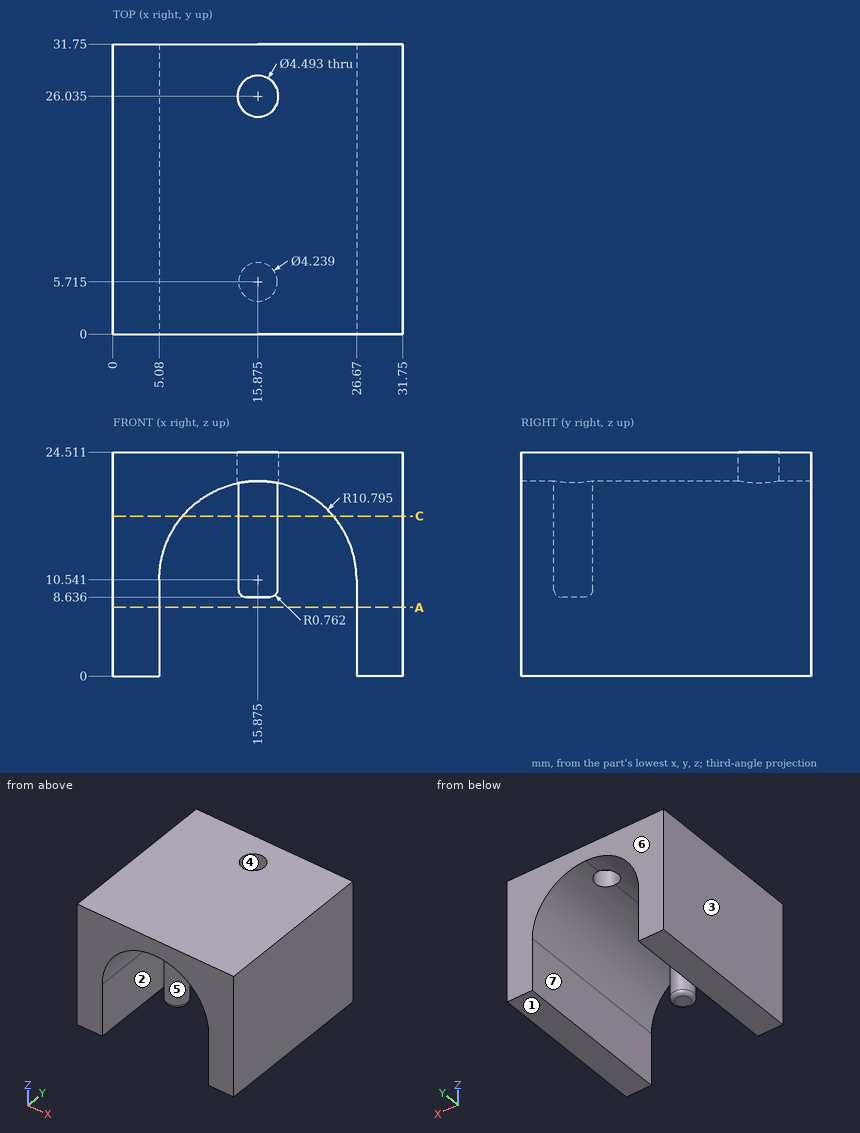
For this review, use the dimensioned drawing (mm, ordinates from the lowest corner) and the shaded views. A direction names the side the tool comes from. Give positions to 0.01 mm unless a question says otherwise; leave off trailing zeros. Write each loop counter-clockwise with the first axis right and the second up, starting at its lowest first coordinate (ties: lowest second). Pieces come first, ordered by that corner, then holes.
(1) Tool access review of the marked faces 5, 6 and 7: name each direction out of +Z, -Z, +X, -X, +Y, -Y from which nothing blocks a thin tool from reaching the whole face with its end or side.
(2) The part is to be moulded in two halves that separate along X. For the marked faces 1, 2, 3 and 4, say which applies: released by +X, released by -X, zero draft, split by the parting line, or undercut.
(3) Consider section A-A, the plane z = 7.5. Give the boundary of the cut face in (x, y).
(4) Consider section C-C, the plane z = 17.5. Give the number of separate pieces and of enclosed holes in the cut face, and give its area (3 significant figures).
(5) For P1, Ø1.5, axis at y = 18, z = 21.5, coming from the -X side; P2, Ø0.8, axis at x = 16, y = 6, coming from the -Z side; P3, Ø10, axis at x = 12.5, z = 14, coming from the -Y side, all flat-tipped, find the tip position at first contact; note any pin that passes through.
(6) To check wall thickness, follow L1, parallel to X at y = 16, z = 2; L2, parallel to X at y = 29.5, z = 18.25; L3, parallel to Z at x = 16, y = 9 (1 decimal). State the ranges of each line that lie inside material, in increasing order.
Returned:
1. face 5: -Z
1. face 6: +Z, -Z, +X, -X, +Y
1. face 7: -Z, +Y, -Y
2. face 1: zero draft
2. face 2: undercut
2. face 3: released by -X
2. face 4: undercut
3. outline: (0, 0) - (5.08, 0) - (5.08, 31.75) - (0, 31.75) - close; (26.67, 0) - (31.75, 0) - (31.75, 31.75) - (26.67, 31.75) - close
4. separate pieces: 3
4. enclosed holes: 0
4. area: 498 mm2
5. P1: stops at x = 0
5. P2: stops at z = 8.64
5. P3: stops at y = 3.6
6. L1: x = 0 to 5.08, 26.67 to 31.75
6. L2: x = 0 to 8.32, 23.43 to 31.75
6. L3: z = 21.3 to 24.5
